Work out the finished part from the listing and answer in its coordinate system (mm). A direction names the side the tool comes from. Coordinates: 2 decimals unless noted, no trailing zeros. Write each loop counter-clockwise with the first axis right and the second up, starting at its lowest first coordinate (ties: lowest second). Pieces come first, ordered by that corner, then holes. Notation, with made-up numbers: (71.5, -5) - (118.5, -5) arc R37 cw to (118.5, 34) - close; hole circle Ø9 at (79.25, 76.25). An arc over 180 degrees is marked (long way). Answer as a JSON object with one key per item and string values. Group by question number.
from build123d import *

# Parameters (mm, degrees)
BOSS_EXTRUDE1_DEPTH = 3
SKETCH2_R           = 1.75
CUT_EXTRUDE1_DEPTH  = 4
FILLET1_R           = 1.5
FILLET3_R           = 3
FILLET2_R           = 1


with BuildPart() as part:
    # Sketch1 → Boss-Extrude1 (new body)
    with BuildSketch(Plane(origin=(0, 0, 0), x_dir=(1, 0, 0), z_dir=(0, 1, 0))):
        with BuildLine():
            Line((-12.491196746, 15), (-4.491196746, 15))
            Line((-4.491196746, 15), (-4.491196746, 8))
            Line((-4.491196746, 8), (13.75, 8))
            Line((13.75, 8), (13.75, -8))
            Line((13.75, -8), (-4.491196746, -8))
            Line((-4.491196746, -8), (-4.491196746, -15))
            Line((-4.491196746, -15), (-12.491196746, -15))
            ThreePointArc((-12.491196746, -15), (-13.75, 0), (-12.491196746, 15))
        make_face()
    extrude(amount=BOSS_EXTRUDE1_DEPTH)

    # Sketch2 → Cut-Extrude1 (cut, through all)
    with BuildSketch(Plane(origin=(0, 3, 0), x_dir=(1, 0, 0), z_dir=(0, 1, 0))):
        with Locations((-9.25, 11)):
            Circle(SKETCH2_R)
    cut_extrude1 = extrude(amount=-CUT_EXTRUDE1_DEPTH, mode=Mode.SUBTRACT)

    # Mirror1: Cut-Extrude1 across plane
    add(cut_extrude1.mirror(Plane.XY), mode=Mode.SUBTRACT)

    # Fillet1
    fillet1_edges = [part.edges().sort_by_distance(p)[0] for p in [
        (-4.491196746, 1.5, -8),
        (13.75, 1.5, -8),
        (13.75, 1.5, 8),
        (-4.491196746, 1.5, 8),
    ]]
    fillet(fillet1_edges, radius=FILLET1_R)

    # Fillet3
    fillet3_edges = [part.edges().sort_by_distance(p)[0] for p in [
        (-4.491196746, 1.5, -15),
        (-4.491196746, 1.5, 15),
    ]]
    fillet(fillet3_edges, radius=FILLET3_R)

    # Fillet2
    fillet2_edges = [part.edges().sort_by_distance(p)[0] for p in [
        (-4.491196746, 3, -10.75),
        (4.629401627, 3, -8),
        (4.629401627, 3, 8),
        (13.75, 3, 0),
        (13.310660172, 3, 7.560660172),
        (13.310660172, 3, -7.560660172),
        (-4.051856918, 3, -8.439339828),
        (-4.051856918, 3, 8.439339828),
        (-9.991196746, 3, -15),
        (-4.491196746, 3, 10.75),
        (-5.369876403, 3, 14.121320344),
        (-5.369876403, 3, -14.121320344),
        (-9.991196746, 3, 15),
    ]]
    fillet(fillet2_edges, radius=FILLET2_R)


solid = part.part
Q1. Section D-D on x = 10.5 is taken. Determine the outline of the cut face in (y, z), plus the area to 3 significant figures.
Q2. Section A-A on x = -9.25 is taken. Determine the outline of the cut face in (y, z), plus the area to 3 significant figures.
Q3. Section B-B on y = 1.6 is taken. Determine the outline of the cut face in (x, z).
Q4. A tool of negligible diameter and unlimited length cuts with its end or side. For faces 4 (the face through (-10, 1, -15)), 5 (the face through (4.736, 2.699, -7.715)), 6 (the face through (5, 1, -8)), 7 (the face through (-4.776, 2.699, 10.768)), 8 (the face through (5, 1, 8)), from which of +Z, -Z, +X, -X, +Y, -Y can it reach the whole face along a straight path? Write none if from no direction.
Q5. Section C-C on z = -10 is taken. Determine the outline of the cut face in (x, y), plus the area to 3 significant figures.
Q6. Flat-ended cylindrical pins translate along their axes: pin 1 Ø1 at (x, y) = (3, 1) entering from -Z; pin 2 Ø2 at (x, z) = (-9.25, -11) entering from -Y; pin 3 Ø0.6 at (x, y) = (7, 1) entering from +Z; pin 4 Ø1.6 at (y, z) = (1, 10.5) entering from +X. Find the tip coordinate at first contact, or state that the pin passes through.
Q7. Consider L1, parallel to Z at x = -9.25, y = 0.9; L2, parallel to X at y = 1.95, z = 11; L3, parallel to X at y = 2.7, z = 12. Determine where each line is inside the solid, lowest interval first. Write a range as from..to.
Q8. For a pull along Z with two mould halves and no side action, classify faces 1 (the face through (-4.06, 1.01, 8.45)), 2 (the face through (-13.75, 1.48, 0.21)), 3 (the face through (-8.309, 1.521, 12.476)) as +Z half, -Z half, draft (parallel to the pull), parting line (faces both ways), or undercut.
Numbers:
{
 "1": {"outline": "(0, -8) - (2, -8) arc R1 ccw to (3, -7) - (3, 7) arc R1 ccw to (2, 8) - (0, 8) - close", "area": "47.6 mm²"},
 "2": {"outline": "(0, -15) - (2, -15) arc R1 ccw to (3, -14) - (3, -12.75) - (0, -12.75) - close; (0, -9.25) - (3, -9.25) - (3, 9.25) - (0, 9.25) - close; (0, 12.75) - (3, 12.75) - (3, 14) arc R1 ccw to (2, 15) - (0, 15) - close", "area": "68.6 mm²"},
 "3": {"outline": "(-12.49, -15) - (-7.49, -15) arc R3 ccw to (-4.49, -12) - (-4.49, -9.5) arc R1.5 cw to (-2.99, -8) - (12.25, -8) arc R1.5 ccw to (13.75, -6.5) - (13.75, 6.5) arc R1.5 ccw to (12.25, 8) - (-2.99, 8) arc R1.5 cw to (-4.49, 9.5) - (-4.49, 12) arc R3 ccw to (-7.49, 15) - (-12.49, 15) arc R90 ccw to start; hole circle Ø3.5 at (-9.25, -11); hole circle Ø3.5 at (-9.25, 11)"},
 "4": {"face 4": "-Z, +X, -X, +Y, -Y", "face 5": "-Z, +X, +Y", "face 6": "-Z, +X, +Y, -Y", "face 7": "+Z, +X, +Y", "face 8": "+Z, +X, +Y, -Y"},
 "5": {"outline": "(-13.19, 0) - (-10.69, 0) - (-10.69, 3) - (-13.19, 3) - close; (-7.81, 0) - (-4.49, 0) - (-4.49, 2) arc R1 ccw to (-5.49, 3) - (-7.81, 3) - close", "area": "17.3 mm²"},
 "6": {"pin 1": "stops at z = -8", "pin 2": "passes through", "pin 3": "stops at z = 8", "pin 4": "stops at x = -4.49"},
 "7": {"L1": "z = -15..-12.75, -9.25..9.25, 12.75..15", "L2": "x = -13.08..-11, -7.5..-4.49", "L3": "x = -12.95..-10.69, -7.81..-4.78"},
 "8": {"face 1": "+Z half", "face 2": "parting line", "face 3": "undercut"}
}
